Can you work these out from the model? Positions are in its coordinate system, mm. A direction names the side the tool comes from. Give positions to 0.01 mm unless a question says otherwise; leave off trailing zeros. Order: outer loops, then holes, each group sorted by start corner. A loop starts at its lowest first (then second) coordinate and runs counter-clockwise, first axis right, second up. Notation, with made-up numbers: M 59.25,67.25 L 87.25,67.25 A21 cw 87.25,101.25 Z; hole C 44,21 d3. An arc over 180 degrees is marked long. One line per question, with ' | ' between items. Start each with the question number.
1) If we section it at C-C, the plane x = 7.5: Please give me the cut outline in (y, z), plus the area to 3 significant figures.
2) If we section it at B-B, the plane y = 37: Please give me the cut outline in (x, z), plus the area to 3 significant figures.
3) If we section it at D-D, the plane x = 18: Please give me the cut outline in (y, z).
4) I'm going to push flat-ended pins straight in: pin 1 Ø8.5 at (x, y) = (5, 18.5) entering from +Z; pin 2 Ø1.8 at (y, z) = (22, 23) entering from -X; pin 3 Ø4.5 at (x, z) = (-23.5, 13.5) entering from +Y; pin 4 Ø4 at (x, y) = (0, 24.5) entering from -Z. Where does each tip first touch, or does it pass through?
5) For faces 5 (the flat face through (-26.33, 6, 13)), 6 (the flat face through (-22, 2.874, 9)), 7 (the flat face through (-17.801, 33, 13)), 8 (the flat face through (3, 22, 0)), 9 (the flat face through (2, 31, 21.715)), which set-ups out of +Z, -Z, +X, -X, +Y, -Y let a thin tool reach every point of the face, with its end or its side?
6) Thinking about a two-plate mould opening in Y: for faces 1 (the flat face through (-12, 33, 25.4)), 2 (the cylindrical face through (-6.966, 11.273, 11.765)), 3 (the flat face through (3.35, -2.8, 12.52)), 4 (the cylindrical face through (10.01, 11.27, 11.77)), which applies, +Y half, -Y half, draft (parallel to the pull), parting line (faces both ways), or undercut?
7) If we section it at A-A, the plane z = 23.25: Please give me the cut outline in (x, y), plus the area to 3 significant figures.
8) Please list where these lines run through material, in increasing order: line 1 along X through (y, z) = (-6.5, 3.5); line 2 along Y through (x, z) = (-23, 16.25); line 3 along X through (y, z) = (15.5, 14.5). Write a range as [from, to].
```python
from build123d import *

# Parameters (mm, degrees)
F1_W     = 8.5294544697
F1_H     = 5.7481119875
F2_DEPTH = 25.4
F4_DEPTH = 48.0255407671
F5_W     = 16.9233079068
F5_H     = 3.6851934433
F6_DEPTH = 69.7200267965
F7_R     = 4.0401840977
F7_R_2   = 4.3013200875
F7_R_3   = 4.1544186405
F7_R_4   = 3.7387935899
F8_DEPTH = 52.7287156055


with BuildPart() as f2:
    # F1 (on face) → F2 (new body)
    with BuildSketch(Plane.XY):
        Polygon((21.6944832355, -13.6285861954), (21.6944832355, 56.0904406011), (-17.8006030619, 56.0904406011), (-17.8006030619, 8.622167632), (-17.8006030619, 2.8740556445), (-17.8006030619, -13.6285861954), align=None)
        with Locations((-22.0653302968, 5.7481116382)):
            Rectangle(F1_W, F1_H)
    extrude(amount=F2_DEPTH)

    # F3 (on face) → F4 (cut, through all)
    with BuildSketch(Plane.YZ.offset(21.6944832355)):
        Polygon((-13.6285861954, 25.4), (-13.6285861954, 0), (8.3440328017, 25.4), align=None)
    extrude(amount=-F4_DEPTH, mode=Mode.SUBTRACT)

    # F5 (on face) → F6 (cut, through all)
    with BuildSketch(Plane(origin=(0, 56.0904406011, 0), x_dir=(-1, 0, 0), z_dir=(0, 1, 0))):
        with Locations((-2.0361964125, 23.5574032784)):
            Rectangle(F5_W, F5_H)
    extrude(amount=-F6_DEPTH, mode=Mode.SUBTRACT)

    # F7 (on face) → F8 (cut, through all)
    with BuildSketch(Plane(origin=(0, -7.7951788741, 6.7433265912), x_dir=(1, 0, 0), z_dir=(0, -0.7562887497, 0.6542379744))):
        with Locations((-6.4254575409, 0)):
            Circle(F7_R)
        with Locations((10.4978503659, 0)):
            Circle(F7_R_2)
        with Locations((-6.4254575409, 12.1534615755)):
            Circle(F7_R_3)
        with Locations((10.4978503659, 12.5690866262)):
            Circle(F7_R_4)
    extrude(amount=-F8_DEPTH, mode=Mode.SUBTRACT)


solid = f2.part
```
Results found:
1) outline: M -13.63,0 L -4.71,0 L -9.81,4.41 Z; M -5.78,9.08 L 4.71,0 L 15.8,0 L -1.03,14.56 Z; M 1.89,17.94 L 22.63,0 L 56.09,0 L 56.09,21.71 L 5.16,21.71 Z | area: 1,140 mm²
2) outline: M -17.8,0 L 21.69,0 L 21.69,25.4 L 10.5,25.4 L 10.5,21.71 L -6.43,21.71 L -6.43,25.4 L -17.8,25.4 Z | area: 941 mm²
3) outline: M -13.63,0 L 56.09,0 L 56.09,25.4 L 8.34,25.4 Z
4) pin 1: stops at z = 21.71 | pin 2: stops at x = -17.8 | pin 3: stops at y = 8.62 | pin 4: stops at z = 0
5) face 5: +Z, -Z, -X, +Y, -Y | face 6: +Z, -Z, -X, -Y | face 7: +Z, -Z, -X, +Y | face 8: -Z, +X, -X, +Y, -Y | face 9: +Z, +Y, -Y
6) face 1: draft | face 2: undercut | face 3: -Y half | face 4: undercut
7) outline: M -26.33,6.48 L -6.43,6.48 L -6.43,56.09 L -17.8,56.09 L -17.8,8.62 L -26.33,8.62 Z; M 10.5,6.48 L 21.69,6.48 L 21.69,56.09 L 10.5,56.09 Z | area: 1,140 mm²
8) line 1: x = [-17.8, -10.13], [-2.72, 6.51], [14.49, 21.69] | line 2: y = [2.87, 8.62] | line 3: x = [-17.8, 21.69]
